Model file for the job. Use its own axes, mm. A direction names the side the tool comes from. Coordinates: 2 decimals unless noted, no trailing zeros. Write each loop counter-clockwise with the first axis right and the second up, starting at its lowest first coordinate (ties: lowest second). Pieces come first, ordered by that corner, then holes. Notation, with made-up numbers: M 57.5,-3.5 L 83.5,-3.5 A24 cw 83.5,23.5 Z; hole C 43,59 d9. An arc over 180 degrees is marked long. One line per question, with ' | ' between items. Start each with the question number.
(1) Tool access for faces 5 (the face through (-8, 0, -18)), 6 (the face through (4.48, 5.92, -26.29)): list every direction of +Z, -Z, +X, -X, +Y, -Y with a clear straight run to the whole face (end or side of a thin tool).
(2) Cut at B-B (z = -15.5). Write the cut outline in (x, y), plus the area to 3 significant figures.
(3) Cut at C-C (x = 34.5). Write the cut outline in (y, z).
(4) Cut at A-A (x = 0). Write the cut outline in (y, z), plus the area to 3 significant figures.
(5) Wall check: probe 1 along Y at (x, z) = (-12, -36); probe 2 along X at (y, z) = (48, 0); probe 3 along Y at (x, z) = (-22, -9.5). Give the ranges that are in metal, low to high.
(6) Flat gauge pins, fed straight in: pin 1 Ø16.5 at (x, z) = (0, 0) entering from -Y; pin 2 Ø3 at (y, z) = (8, -23) entering from -X; pin 3 Ø1.2 at (y, z) = (5, -21.5) entering from +X; pin 4 Ø2 at (x, z) = (-29, -30) entering from +Y. Where does each tip first touch, or does it go through?
(7) Cut at D-D (y = 47). Write the cut outline in (x, z), plus the area to 3 significant figures.
(8) Two-plate mould, pull along Z, no slides. Class faces 1 (the face through (23, 6, -2)), 2 (the face through (1, 39.572, 8)), 3 (the face through (0.751, 25.433, 32.075)), 4 (the face through (-26.41, 5.92, -3.91)): +Z half, -Z half, draft (parallel to the pull), parting line (faces both ways), or undercut.
from build123d import *

# Parameters (mm, degrees)
SKETCH1_R           = 40
BOSS_EXTRUDE1_DEPTH = 11.684
SKETCH2_R           = 2.5
BOSS_EXTRUDE2_DEPTH = 27.888000104
SKETCH3_R           = 40
BOSS_EXTRUDE3_DEPTH = 20
FILLET1_R           = 2.54
CUT_EXTRUDE1_REACH  = 84.151
SKETCH4_R           = 6.35


with BuildPart() as part:
    # Sketch1 → Boss-Extrude1 (new body)
    with BuildSketch(Plane(origin=(0, 0, 0), x_dir=(1, 0, 0), z_dir=(0, 1, 0))):
        with Locations(Location((0, 0, 0), (0, 0, 270))):
            Circle(SKETCH1_R)
        with BuildLine():
            ThreePointArc((16.146222613, 10.721189548), (11.392188189, 15.680001858), (5.207, 18.669))
            Line((5.207, 18.669), (5.207, 27.051))
            Line((5.207, 27.051), (-5.207, 27.051))
            Line((-5.207, 27.051), (-5.207, 18.669))
            ThreePointArc((-5.207, 18.669), (-11.392188189, 15.680001858), (-16.146222613, 10.721189548))
            Line((-16.146222613, 10.721189548), (-24.117978333, 13.311369995))
            Line((-24.117978333, 13.311369995), (-27.336081312, 3.407067434))
            Line((-27.336081312, 3.407067434), (-19.364325592, 0.816886988))
            ThreePointArc((-19.364325592, 0.816886988), (-18.432947696, -5.989227766), (-15.185914365, -12.042940459))
            Line((-15.185914365, -12.042940459), (-20.112730349, -18.824120906))
            Line((-20.112730349, -18.824120906), (-11.68762737, -24.945316524))
            Line((-11.68762737, -24.945316524), (-6.760811385, -18.164136077))
            ThreePointArc((-6.760811385, -18.164136077), (0, -19.381548184), (6.760811385, -18.164136077))
            Line((6.760811385, -18.164136077), (11.68762737, -24.945316524))
            Line((11.68762737, -24.945316524), (20.112730349, -18.824120906))
            Line((20.112730349, -18.824120906), (15.185914365, -12.042940459))
            ThreePointArc((15.185914365, -12.042940459), (18.432947696, -5.989227766), (19.364325592, 0.816886988))
            Line((19.364325592, 0.816886988), (27.336081312, 3.407067434))
            Line((27.336081312, 3.407067434), (24.117978333, 13.311369995))
            Line((24.117978333, 13.311369995), (16.146222613, 10.721189548))
        make_face(mode=Mode.SUBTRACT)
    extrude(amount=BOSS_EXTRUDE1_DEPTH)

    # Sketch2 → Boss-Extrude2 (add)
    with BuildSketch(Plane(origin=(0, 11.684, 0), x_dir=(1, 0, 0), z_dir=(0, 1, 0))):
        with Locations(Location((-17.45179914, 24.020340816, 0), (0, 0, 270))):
            Circle(SKETCH2_R)
        with Locations(Location((17.45179914, 24.020340816, 0), (0, 0, 270))):
            Circle(SKETCH2_R)
        with Locations(Location((0, -29.690774092, 0), (0, 0, 270))):
            Circle(SKETCH2_R)
    extrude(amount=BOSS_EXTRUDE2_DEPTH)

    # Sketch3 → Boss-Extrude3 (add)
    with BuildSketch(Plane(origin=(0, 39.572000104, 0), x_dir=(1, 0, 0), z_dir=(0, 1, 0))):
        with Locations(Location((0, 0, 0), (0, 0, 270))):
            Circle(SKETCH3_R)
    extrude(amount=BOSS_EXTRUDE3_DEPTH)

    # Fillet1
    fillet1_edges = [part.edges().sort_by_distance(p)[0] for p in [
        (5.207, 5.842, -18.669),
        (5.207, 5.842, -27.051),
        (-5.207, 5.842, -27.051),
        (-5.207, 5.842, -18.669),
        (-16.146222613, 5.842, -10.721189548),
        (-24.117978333, 5.842, -13.311369995),
        (-27.336081312, 5.842, -3.407067434),
        (-19.364325592, 5.842, -0.816886988),
        (-15.185914365, 5.842, 12.042940459),
        (-20.112730349, 5.842, 18.824120906),
        (-11.68762737, 5.842, 24.945316524),
        (-6.760811385, 5.842, 18.164136077),
        (6.760811385, 5.842, 18.164136077),
        (11.68762737, 5.842, 24.945316524),
        (20.112730349, 5.842, 18.824120906),
        (15.185914365, 5.842, 12.042940459),
        (19.364325592, 5.842, -0.816886988),
        (27.336081312, 5.842, -3.407067434),
        (24.117978333, 5.842, -13.311369995),
        (16.146222613, 5.842, -10.721189548),
    ]]
    fillet(fillet1_edges, radius=FILLET1_R)

    # Sketch4 → Cut-Extrude1 (cut, up to next)
    with BuildSketch(Plane(origin=(0, 59.572000104, 0), x_dir=(1, 0, 0), z_dir=(0, 1, 0)), mode=Mode.PRIVATE) as cut_extrude1_sk1:
        with Locations(Location((0, 0, 0), (0, 0, 270))):
            Circle(SKETCH4_R)
    cut_extrude1_tool1 = extrude(cut_extrude1_sk1.sketch, amount=-CUT_EXTRUDE1_REACH, mode=Mode.PRIVATE) & part.part
    add(cut_extrude1_tool1.solids().sort_by_distance((0, 59.572, 0))[0], mode=Mode.SUBTRACT)


solid = part.part
Filled in:
1) face 5: +Z, -Z, +X, -X, -Y | face 6: -Y
2) outline: M -36.87,0 L -11.64,0 L -11.64,11.68 L -36.87,11.68 Z; M -36.87,39.57 L 36.87,39.57 L 36.87,59.57 L -36.87,59.57 Z; M 11.64,0 L 36.87,0 L 36.87,11.68 L 11.64,11.68 Z | area: 2,060 mm²
3) outline: M 0,-20.24 L 11.68,-20.24 L 11.68,20.24 L 0,20.24 Z; M 39.57,-20.24 L 59.57,-20.24 L 59.57,20.24 L 39.57,20.24 Z
4) outline: M 0,-40 L 11.68,-40 L 11.68,-27.05 L 0,-27.05 Z; M 0,19.38 L 11.68,19.38 L 11.68,27.19 L 39.57,27.19 L 39.57,6.35 L 59.57,6.35 L 59.57,40 L 39.57,40 L 39.57,32.19 L 11.68,32.19 L 11.68,40 L 0,40 Z; M 39.57,-40 L 59.57,-40 L 59.57,-6.35 L 39.57,-6.35 Z | area: 1,880 mm²
5) probe 1: 0 to 11.68, 39.57 to 59.57 | probe 2: -40 to -6.35, 6.35 to 40 | probe 3: 39.57 to 59.57
6) pin 1: y = 39.57 | pin 2: x = -33.73 | pin 3: x = 34.11 | pin 4: through
7) outline: C 0,0 d80; hole C 0,0 d12.7 | area: 4,900 mm²
8) face 1: undercut | face 2: draft | face 3: parting line | face 4: undercut
